Here's how the part is built. I have some questions about the finished solid (model axes, mm). Round coordinates to 2 decimals unless told otherwise and drop trailing zeros. Loops run counter-clockwise (first coordinate to the right, second up) from the corner with the lowest first, then second, coordinate; pieces in that order, holes last. Notation, with made-up numbers: (37.5, -10.75) - (63.5, -10.75) arc R23 ccw to (63.5, 4.25) - close; hole circle Ø1 at (50.25, 40). An arc over 180 degrees is marked (long way). Answer as a JSON object with one key per item and string values. Group by question number.
1) If I drill on line 1 along Y through (x, z) = (0, 0.35); line 2 along X through (y, z) = (0, 0.75); line 3 along Y through (x, z) = (-2, 0.3), over which ranges is the centre line in solid material (lowest first)? Write a range as [from, to].
2) I want a section at B-B, the plane y = 0. Please give me the cut outline in (x, z).
3) I want a section at D-D, the plane x = -1.5. Please give me the cut outline in (y, z), then the cut area to 3 significant figures.
4) I want a section at A-A, the plane x = 0. Please give me the cut outline in (y, z).
5) I want a section at C-C, the plane z = 0.25. Please give me the cut outline in (x, y), then the cut area to 3 significant figures.
6) If we mould it in two halves opening along Y, with no side actions, what happens to faces 1 (the face through (-5, 0.1, 0.5)), 2 (the face through (-3.1, -0.1, 0.5)), 3 (the face through (-4, 0, 0))? For each: pulls with the +Y half, pulls with the -Y half, needs draft (parallel to the pull), parting line crosses it, or undercut.
from build123d import *

# Parameters (mm, degrees)
BOSS_EXTRUDE1_DEPTH = 0.95
FILLET1_R           = 2


with BuildPart() as part:
    # Sketch1 → Boss-Extrude1 (new body)
    with BuildSketch(Plane.XY):
        with BuildLine():
            Line((1.546099973, 2.686926659), (2.493709634, 4.333752676))
            ThreePointArc((2.493709634, 4.333752676), (-4.999994729, -0.007260445), (2.506285094, -4.326492231))
            Line((2.506285094, -4.326492231), (1.553896759, -2.682425183))
            ThreePointArc((1.553896759, -2.682425183), (-3.099996732, -0.004501476), (1.546099973, 2.686926659))
        make_face()
    extrude(amount=BOSS_EXTRUDE1_DEPTH)

    # Fillet1
    fillet1_edges = [part.edges().sort_by_distance(p)[0] for p in [
        (1.546099973, 2.686926659, 0.475),
        (1.553896759, -2.682425183, 0.475),
    ]]
    fillet(fillet1_edges, radius=FILLET1_R)


solid = part.part
Outcome:
{
 "1": {"line 1": "[-5, -3.1], [3.1, 5]", "line 2": "[-5, -3.1]", "line 3": "[-4.58, -2.37], [2.37, 4.58]"},
 "2": {"outline": "(-5, 0) - (-3.1, 0) - (-3.1, 0.95) - (-5, 0.95) - close"},
 "3": {"outline": "(-4.77, 0) - (-2.71, 0) - (-2.71, 0.95) - (-4.77, 0.95) - close; (2.71, 0) - (4.77, 0) - (4.77, 0.95) - (2.71, 0.95) - close", "area": "3.91 mm^2"},
 "4": {"outline": "(-5, 0) - (-3.1, 0) - (-3.1, 0.95) - (-5, 0.95) - close; (3.1, 0) - (5, 0) - (5, 0.95) - (3.1, 0.95) - close"},
 "5": {"outline": "(0.37, 3.08) arc R2 ccw to (2.34, 4.07) - (2.49, 4.33) arc R5 ccw (long way) to (2.51, -4.33) - (2.35, -4.06) arc R2 ccw to (0.38, -3.08) arc R3.1 cw (long way) to start", "area": "31.4 mm^2"},
 "6": {"face 1": "parting line crosses it", "face 2": "undercut", "face 3": "needs draft"}
}
